```python
from build123d import *

# Parameters (mm, degrees)
F0_W     = 35
F0_H     = 100
F1_DEPTH = 30
F2_R     = 15.15
F3_DEPTH = 999
F4_R     = 4.15
F5_DEPTH = 25


with BuildPart() as f1:
    # F0 (on Top) → F1 (new body)
    with BuildSketch(Plane.XY):
        with Locations((17.5, 50)):
            Rectangle(F0_W, F0_H)
    extrude(amount=F1_DEPTH)

    # F2 (on face) → F3 (cut)
    with BuildSketch(Plane.XZ):
        with Locations((17.5, 30)):
            Circle(F2_R)
    extrude(amount=-F3_DEPTH, mode=Mode.SUBTRACT)

    # F4 (on face) → F5 (cut)
    with BuildSketch(Plane(origin=(0, 0, 0), x_dir=(1, 0, 0), z_dir=(0, 0, -1))):
        with Locations((17.5, -50)):
            Circle(F4_R)
    extrude(amount=-F5_DEPTH, mode=Mode.SUBTRACT)


solid = f1.part
```
Check sheet for the modelled part. Datum: model origin and axes. Units: mm. Round coordinates to 2 decimals unless told otherwise and drop trailing zeros. Loops run counter-clockwise (first coordinate to the right, second up) from the corner with the lowest first, then second, coordinate; pieces in that order, holes last. Notation, with made-up numbers: M 57.5,2 L 89.5,2 A21 cw 89.5,40 Z; hole C 73,23 d1. An arc over 180 degrees is marked long. Answer as a JSON object with one key per item and string values.
1. Scan lines: line 1 (X direction, y = 50, z = 11.25); line 2 (Y direction, x = 17.5, z = 6); line 3 (X direction, y = 68, z = 27). Record each from-to range of solid material in increasing order.
Reply:
{"line 1": "x = 0 to 13.35, 21.65 to 35", "line 2": "y = 0 to 45.85, 54.15 to 100", "line 3": "x = 0 to 2.65, 32.35 to 35"}
2. Section check B-B (y = 50). Record the boundary of the cut face in (x, z), plus the area to 3 significant figures.
Reply:
{"outline": "M 0,0 L 13.35,0 L 13.35,15.43 A15.15 cw 2.35,30 L 0,30 Z; M 21.65,0 L 35,0 L 35,30 L 32.65,30 A15.15 cw 21.65,15.43 Z", "area": "565 mm²"}
3. Mould release check, pull along X, two halves, no side actions. Record for faces 1 (the cylindrical face through (16.96, 45.885, 7.607)), 2 (the flat face through (35, 49, 15)), 3 (the flat face through (17, 0, 11)): pulls with the +X half, pulls with the -X half, needs draft (parallel to the pull), parting line crosses it, or undercut.
Reply:
{"face 1": "undercut", "face 2": "pulls with the +X half", "face 3": "needs draft"}
4. Section check A-A (x = 17.5). Record the boundary of the cut face in (y, z).
Reply:
{"outline": "M 0,0 L 45.85,0 L 45.85,14.85 L 0,14.85 Z; M 54.15,0 L 100,0 L 100,14.85 L 54.15,14.85 Z"}
5. Gauge pin test, flat ends, axial feed: P1, Ø6, axis at x = 6.5, z = 24, coming from the +Y side; P2, Ø9.5, axis at x = 17.5, y = 50, coming from the +Z side; P3, Ø4, axis at x = 7.5, y = 41.5, coming from the +Z side. Record the tip position at first contact, or that the pin passes through.
Reply:
{"P1": "stops at y = 100", "P2": "stops at z = 15.61", "P3": "stops at z = 20.75"}
6. Section check C-C (z = 9). Record the boundary of the cut face in (x, y).
Reply:
{"outline": "M 0,0 L 35,0 L 35,100 L 0,100 Z; hole C 17.5,50 d8.3"}
7. Section check D-D (z = 18.5). Record the boundary of the cut face in (x, y).
Reply:
{"outline": "M 0,0 L 7.64,0 L 7.64,100 L 0,100 Z; M 27.36,0 L 35,0 L 35,100 L 27.36,100 Z"}
